Geometry check sheet. Reference: the model listing, model coordinates, mm. Face numbers are marked on the shaded views. Coordinates: 2 decimals unless noted, no trailing zeros. Write each loop counter-clockwise with the first axis right and the second up, starting at its lowest first coordinate (ties: lowest second). Pieces come first, ordered by that corner, then holes. Notation, with made-up numbers: (72, 18) -> (113, 18) arc R35 cw to (113, 50) -> close; hole circle Ø8 at (-16.75, -25.75). An arc over 180 degrees is marked (long way). One line per question, with ' | ' between items.
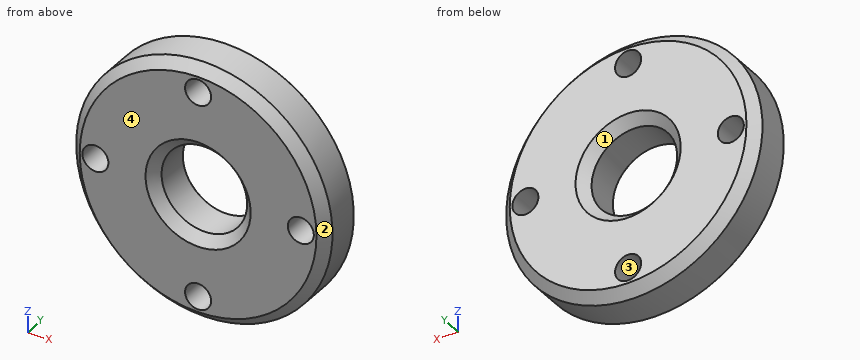
from build123d import *

# Parameters (mm, degrees)
SKETCH1_R           = 33.274
SKETCH1_R_2         = 11.1125
SKETCH1_R_3         = 3.3782
BOSS_EXTRUDE1_DEPTH = 13.716
CHAMFER1_SIZE       = 2.54


with BuildPart() as part:
    # Sketch1 → Boss-Extrude1 (new body)
    with BuildSketch(Plane(origin=(0, 0, 0), x_dir=(1, 0, 0), z_dir=(0, 1, 0))):
        with Locations(Location((0, 0, 0), (0, 0, 270))):
            Circle(SKETCH1_R)
        with Locations(Location((0, 0, 0), (0, 0, 270))):
            Circle(SKETCH1_R_2, mode=Mode.SUBTRACT)
        with Locations(Location((0, 26.67, 0), (0, 0, 270))):
            Circle(SKETCH1_R_3, mode=Mode.SUBTRACT)
        with Locations(Location((26.67, 0, 0), (0, 0, 270))):
            Circle(SKETCH1_R_3, mode=Mode.SUBTRACT)
        with Locations(Location((0, -26.67, 0), (0, 0, 270))):
            Circle(SKETCH1_R_3, mode=Mode.SUBTRACT)
        with Locations(Location((-26.67, 0, 0), (0, 0, 270))):
            Circle(SKETCH1_R_3, mode=Mode.SUBTRACT)
    extrude(amount=BOSS_EXTRUDE1_DEPTH)

    # Chamfer1
    chamfer1_edges = [part.edges().sort_by_distance(p)[0] for p in [
        (0, 0, -33.274),
        (0, 13.716, -33.274),
        (0, 0, -11.1125),
        (0, 13.716, -11.1125),
    ]]
    chamfer(chamfer1_edges, length=CHAMFER1_SIZE)


solid = part.part
1. Cross-section at B-B on x = 0. Record the boundary of the cut face in (y, z), and give its area (3 significant figures).
Worked answers:
outline: (0, -30.73) -> (2.54, -33.27) -> (11.18, -33.27) -> (13.72, -30.73) -> (13.72, -30.05) -> (0, -30.05) -> close; (0, -23.29) -> (13.72, -23.29) -> (13.72, -13.65) -> (11.18, -11.11) -> (2.54, -11.11) -> (0, -13.65) -> close; (0, 13.65) -> (2.54, 11.11) -> (11.18, 11.11) -> (13.72, 13.65) -> (13.72, 23.29) -> (0, 23.29) -> close; (0, 30.05) -> (13.72, 30.05) -> (13.72, 30.73) -> (11.18, 33.27) -> (2.54, 33.27) -> (0, 30.73) -> close | area: 397 mm²
2. Cross-section at A-A on z = 0. Record the boundary of the cut face in (x, y), and give its area (3 significant figures).
Worked answers:
outline: (-33.27, 2.54) -> (-30.73, 0) -> (-30.05, 0) -> (-30.05, 13.72) -> (-30.73, 13.72) -> (-33.27, 11.18) -> close; (-23.29, 0) -> (-13.65, 0) -> (-11.11, 2.54) -> (-11.11, 11.18) -> (-13.65, 13.72) -> (-23.29, 13.72) -> close; (11.11, 2.54) -> (13.65, 0) -> (23.29, 0) -> (23.29, 13.72) -> (13.65, 13.72) -> (11.11, 11.18) -> close; (30.05, 0) -> (30.73, 0) -> (33.27, 2.54) -> (33.27, 11.18) -> (30.73, 13.72) -> (30.05, 13.72) -> close | area: 397 mm²
3. Cross-section at C-C on y = 3.5. Record the boundary of the cut face in (x, z) (1 decimal), and give its area (3 significant figures).
Worked answers:
outline: circle Ø66.5 at (0, 0); hole circle Ø6.8 at (-26.7, 0); hole circle Ø22.2 at (0, 0); hole circle Ø6.8 at (0, -26.7); hole circle Ø6.8 at (0, 26.7); hole circle Ø6.8 at (26.7, 0) | area: 2,950 mm²
4. Material ranges on line 1 (X direction, y = 10.5, z = 0); line 2 (X direction, y = 6.75, z = 3); line 3 (Z direction, x = 7.5, y = 2.5), recorded low to high. Write a range as from..to.
Worked answers:
line 1: -33.27..-30.05, -23.29..-11.11, 11.11..23.29, 30.05..33.27 | line 2: -33.14..-28.22, -25.12..-10.7, 10.7..25.12, 28.22..33.14 | line 3: -32.38..-8.25, 8.25..32.38
5. Mould release check, pull along Z, two halves, no side actions. Record for the marked faces 1, 2, 3 and 4: released by +Z, released by -Z, zero draft, split by the parting line, or undercut.
Worked answers:
face 1: undercut | face 2: split by the parting line | face 3: undercut | face 4: zero draft
6. Go/stop test with flat-tipped pins: P1, Ø4, axis at x = 15.5, y = 6.5, coming from the -Z side; P2, Ø9, axis at x = 26.67, z = 0, coming from the +Y side; P3, Ø8, axis at y = 6, z = 8, coming from the +X side; P4, Ø5, axis at x = -17.5, y = 4, coming from the -Z side. Record where each tip stops, or that it passes through.
Worked answers:
P1: z = -30.41 | P2: y = 13.72 | P3: x = 33.03 | P4: z = -29.7
